The listing builds one solid part. Answer for the finished solid, in the listing's coordinates (mm). Face numbers are marked on the shaded views. A direction names the side the tool comes from. Round coordinates to 2 decimals unless told otherwise and drop trailing zeros. Loops run counter-clockwise (first coordinate to the right, second up) from the corner with the lowest first, then second, coordinate; pieces in that order, holes last. Notation, with made-up numbers: (-31.75, 81) -> (-9.75, 81) arc R16 cw to (-9.75, 97) -> close; hole circle Ø3 at (-27, -19). An arc over 180 degrees is marked (long way). Answer in a Markdown table with one row per item. Add a question column.
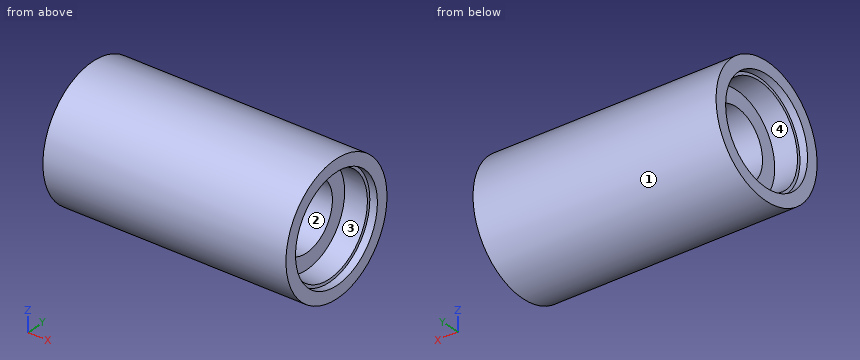
```python
from build123d import *


with BuildPart() as part:
    # Sketch1 → Revolve1 (revolve)
    with BuildSketch(Plane.XY):
        Polygon((0, 21.1), (40, 21.1), (40, 17.1), (37.5, 17.1), (37.5, 16.1), (30, 16.1), (30, 11), (0, 11), align=None)
    revolve1 = revolve(axis=Axis((0, 0, 0), (1, 0, 0)))

    # Mirror1: Revolve1 across plane
    add(revolve1.mirror(Plane(origin=(0, 0, 0), x_dir=(0, 0, 1), z_dir=(1, 0, 0))))


solid = part.part
```
Item 1: Section D-D, the plane x = -34 is taken. Write down the section's boundary in (y, z), and give its area (3 significant figures).
Item 2: Section C-C, the plane y = -15 is taken. Write down the section's boundary in (x, z).
Item 3: Consider L1, parallel to Z at x = -35, y = 0; L2, parallel to Z at x = -11, y = 0; L3, parallel to Z at x = -6.5, y = -18. Determine where each line is inside the solid, lowest interval first. Write a range as from..to.
Item 4: Section A-A, the plane y = 0 is taken. Write down the section's boundary in (x, z), and give its area (3 significant figures).
Item 5: Flat-ended cylindrical pins translate along their axes: P1, Ø5, axis at x = -3, z = 4.5, coming from the -Y side (3 decimals); P2, Ø4, axis at x = 26.5, y = -2, coming from the -Z side; P3, Ø1.5, axis at y = -14.5, z = 3, coming from the +X side; P4, Ø10, axis at y = 5.5, z = -11.5, coming from the -X side. Find the tip coordinate at first contact, or state that the pin passes through.
Item 6: The mould has two halves that part along Y. Classify the marked faces 1 and 2: +Y half, -Y half, draft (parallel to the pull), parting line (faces both ways), or undercut.
Item 7: For the marked faces 3 and 4, determine the directions among +Z, -Z, +X, -X, +Y, -Y from which every point of the face is accessible in a straight line to the end or side of a thin tool.
Here are the results:
| question | item | result |
|---|---|---|
| 1 | outline | circle Ø42.2 at (0, 0); hole circle Ø32.2 at (0, 0) |
| 1 | area | 584 mm² |
| 2 | outline | (-40, -14.84) -> (40, -14.84) -> (40, -8.21) -> (37.5, -8.21) -> (37.5, -5.85) -> (30, -5.85) -> (30, 5.85) -> (37.5, 5.85) -> (37.5, 8.21) -> (40, 8.21) -> (40, 14.84) -> (-40, 14.84) -> (-40, 8.21) -> (-37.5, 8.21) -> (-37.5, 5.85) -> (-30, 5.85) -> (-30, -5.85) -> (-37.5, -5.85) -> (-37.5, -8.21) -> (-40, -8.21) -> close |
| 3 | L1 | z = -21.1..-16.1, 16.1..21.1 |
| 3 | L2 | z = -21.1..-11, 11..21.1 |
| 3 | L3 | z = -11.01..11.01 |
| 4 | outline | (-40, -21.1) -> (40, -21.1) -> (40, -17.1) -> (37.5, -17.1) -> (37.5, -16.1) -> (30, -16.1) -> (30, -11) -> (-30, -11) -> (-30, -16.1) -> (-37.5, -16.1) -> (-37.5, -17.1) -> (-40, -17.1) -> close; (-40, 17.1) -> (-37.5, 17.1) -> (-37.5, 16.1) -> (-30, 16.1) -> (-30, 11) -> (30, 11) -> (30, 16.1) -> (37.5, 16.1) -> (37.5, 17.1) -> (40, 17.1) -> (40, 21.1) -> (-40, 21.1) -> close |
| 4 | area | 1,400 mm² |
| 5 | P1 | stops at y = -21.005 |
| 5 | P2 | stops at z = -21.1 |
| 5 | P3 | stops at x = 30 |
| 5 | P4 | stops at x = -40 |
| 6 | face 1 | parting line |
| 6 | face 2 | undercut |
| 7 | face 3 | +X |
| 7 | face 4 | -X |
